Geometry: see drawing. Coordinates: mm, zero at the bounding-box minimum. A direction names the side the tool comes from. Coordinates: 2 decimals unless noted, no trailing zeros. Order: outer loops, then holes, each group sorted by start corner. A loop starts at its lowest first (then second) coordinate and runs counter-clockwise, first axis right, second up.
Item 1: Ray query, line 1 (Z direction, x = 24, y = 50.5); line 2 (Y direction, x = 35, z = 21.5); line 3 (Y direction, x = 16, z = 20). Return the intervals inside material, ascending.
Item 2: Mould query, pull axis X, two halves, no side actions, for the marked faces 1, 2, 3 and 4. Classes: released by +X, released by -X, zero draft, split by the parting line, or undercut.
Item 3: Section C-C on x = 55. Return the cut outline in (y, z).
Item 4: Reachability of the marked faces 5, 6 and 7 from +Z, -Z, +X, -X, +Y, -Y: full face, straight path, thin tool, end or side. Return the list, or none.
Item 5: Section B-B on y = 30. Return the cut outline in (x, z), then the cut area to 3 significant figures.
Item 6: Section D-D on x = 35. Return the cut outline in (y, z), then the cut area to 4 significant figures.
Item 7: Section A-A on z = 26.5. Return the cut outline in (x, y).
Item 8: Contact query for flat-ended pins moving along their axis: P1, Ø5, axis at x = 67, z = 29, coming from the -Y side; P2, Ø1, axis at x = 53.5, y = 84.5, coming from the +Z side; P3, Ø7.5, axis at x = 10, y = 86, coming from the +Z side. Output: stop coordinate, or through.
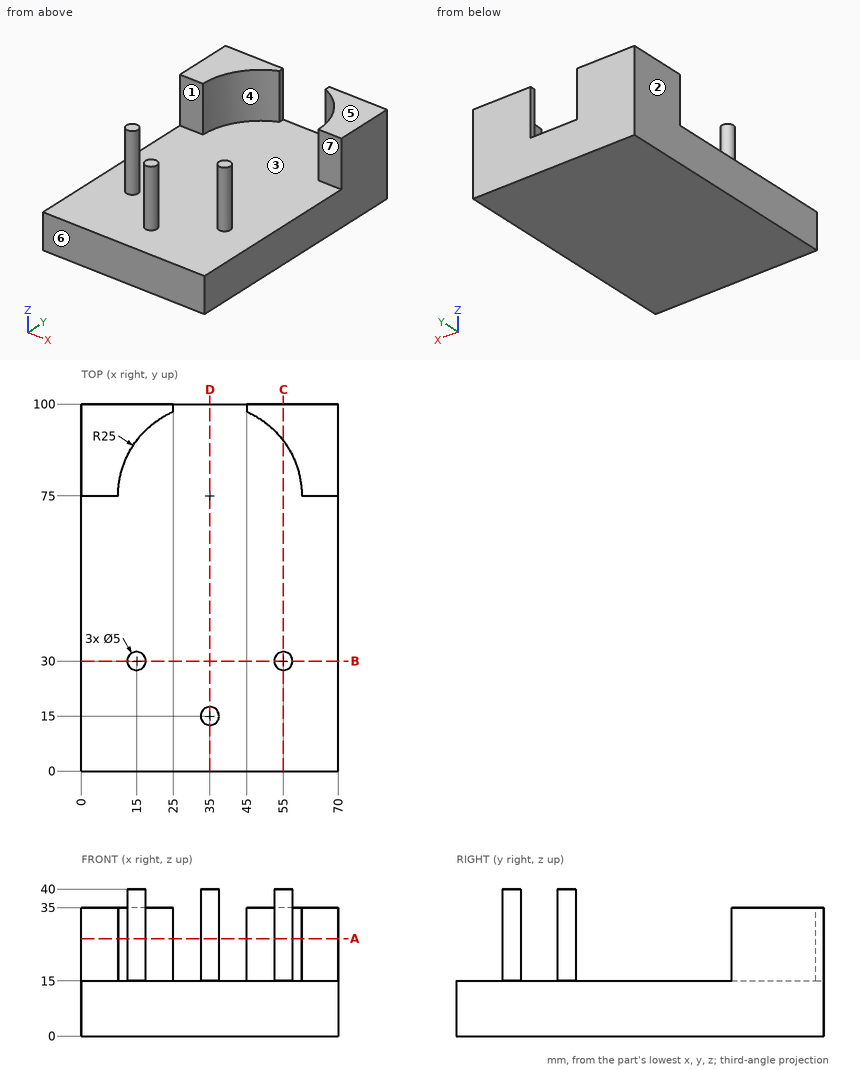
Answer list:
1. line 1: z = 0 to 15
1. line 2: y = 12.5 to 17.5
1. line 3: y = 27.71 to 32.29, 91.25 to 100
2. face 1: zero draft
2. face 2: released by -X
2. face 3: undercut
2. face 4: undercut
3. outline: (0, 0) - (100, 0) - (100, 35) - (90, 35) - (90, 15) - (32.5, 15) - (32.5, 40) - (27.5, 40) - (27.5, 15) - (0, 15) - close
4. face 5: +Z, +X, -X, +Y
4. face 6: +Z, -Z, +X, -X, -Y
4. face 7: +Z, +X, -X, -Y
5. outline: (0, 0) - (70, 0) - (70, 15) - (57.5, 15) - (57.5, 40) - (52.5, 40) - (52.5, 15) - (17.5, 15) - (17.5, 40) - (12.5, 40) - (12.5, 15) - (0, 15) - close
5. area: 1,300 mm2
6. outline: (0, 0) - (100, 0) - (100, 15) - (17.5, 15) - (17.5, 40) - (12.5, 40) - (12.5, 15) - (0, 15) - close
6. area: 1,625 mm2
7. outline: (0, 75) - (10, 75) arc R25 cw to (25, 97.91) - (25, 100) - (0, 100) - close; circle Ø5 at (15, 30); circle Ø5 at (35, 15); (45, 97.91) arc R25 cw to (60, 75) - (70, 75) - (70, 100) - (45, 100) - close; circle Ø5 at (55, 30)
8. P1: stops at y = 75
8. P2: stops at z = 15
8. P3: stops at z = 35
